Geometry: final body of the model. Coordinates: model frame, mm. Face numbers are marked on the shaded views. A direction names the side the tool comes from. Round coordinates to 2 decimals unless told otherwise and drop trailing zeros. Loops run counter-clockwise (first coordinate to the right, second up) from the corner with the lowest first, then second, coordinate; pieces in that order, holes last. Notation, with made-up numbers: M -18.75,-12 L 8.25,-12 A34 ccw 8.25,23 Z; hole C -1.75,71.5 d2. An arc over 180 degrees is marked long. Answer as a JSON object with one key per item and string values.
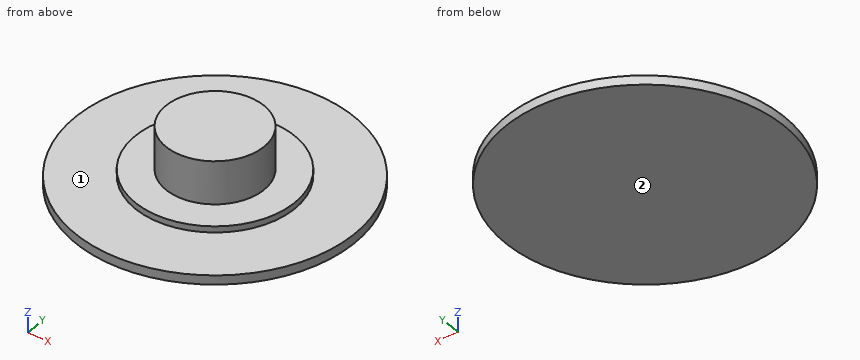
from build123d import *

# Parameters (mm, degrees)
F0_R     = 11.375
F0_R_2   = 6.5
F1_DEPTH = 0.75
F0_R_3   = 4
F2_DEPTH = 1.25
F3_DEPTH = 4.75


with BuildPart() as f1:
    # F0 (on Top) → F1 (new body)
    with BuildSketch(Plane.XY):
        Circle(F0_R)
        Circle(F0_R_2, mode=Mode.SUBTRACT)
    extrude(amount=F1_DEPTH)

    # F0 (on Top) → F2 (join)
    with BuildSketch(Plane.XY):
        Circle(F0_R_2)
        Circle(F0_R_3, mode=Mode.SUBTRACT)
    extrude(amount=F2_DEPTH)

    # F0 (on Top) → F3 (join)
    with BuildSketch(Plane.XY):
        Circle(F0_R_3)
    extrude(amount=F3_DEPTH)


solid = f1.part
1) Ray query, line 1 (Z direction, x = -6.25, y = -7); line 2 (Y direction, x = -8.25, z = 0.35); line 3 (Y direction, x = -3.5, z = 2.5). Return the intervals inside material, ascending.
Results:
{"line 1": "0 to 0.75", "line 2": "-7.83 to 7.83", "line 3": "-1.94 to 1.94"}
2) Reachability of the marked faces 1 and 2 from +Z, -Z, +X, -X, +Y, -Y: full face, straight path, thin tool, end or side. Return the list, or none.
Results:
{"face 1": "+Z", "face 2": "-Z, +X, -X, +Y, -Y"}
3) Section query D-D (x = -4.5). Return the cut outline in (y, z).
Results:
{"outline": "M -10.45,0 L 10.45,0 L 10.45,0.75 L 4.69,0.75 L 4.69,1.25 L -4.69,1.25 L -4.69,0.75 L -10.45,0.75 Z"}
4) Section query A-A (y = 0). Return the cut outline in (x, z) (3 decimals).
Results:
{"outline": "M -11.375,0 L 11.375,0 L 11.375,0.75 L 6.5,0.75 L 6.5,1.25 L 4,1.25 L 4,4.75 L -4,4.75 L -4,1.25 L -6.5,1.25 L -6.5,0.75 L -11.375,0.75 Z"}
5) Section query C-C (z = 0.3). Return the cut outline in (x, y) (3 decimals), and give its area (3 significant figures).
Results:
{"outline": "C 0,0 d22.75", "area": "406 mm2"}
